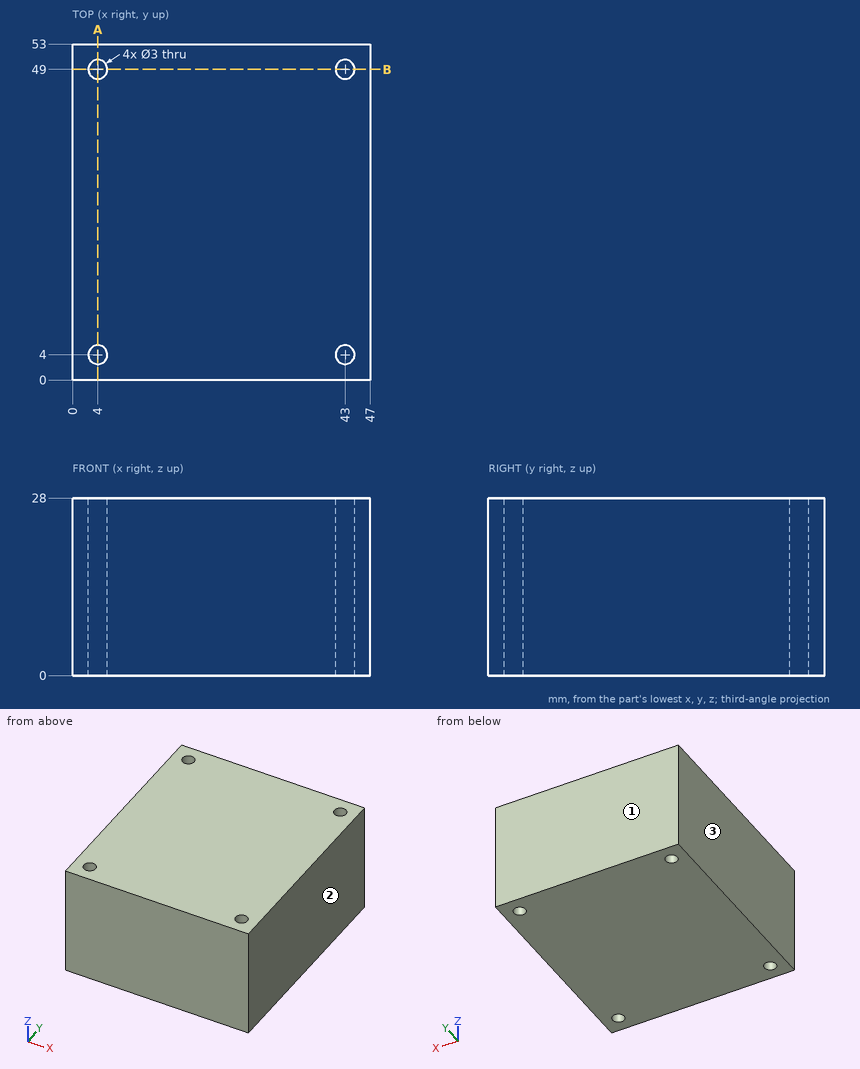
The figure shows three views and two pictorial views of one solid part (mm, origin at its lowest corner). Answer the questions. Give positions to 0.01 mm unless a question says otherwise; leave off trailing zeros. Write each loop counter-clockwise with the first axis right and the second up, starting at its lowest first coordinate (ties: lowest second). Pieces come first, ordered by that corner, then holes. Notation, with made-up numbers: (57, -5) - (85, -5) arc R21 cw to (85, 13) - close; hole circle Ø1 at (17.5, 18). An arc over 180 degrees is marked (long way). Use CSV: the item, a comma, the result in double quotes. Start each with the question number.
Item 1: The mould has two halves that part along X. Classify the marked faces 1, 2 and 3: pulls with the +X half, pulls with the -X half, needs draft (parallel to the pull), parting line crosses it, or undercut.
Item 2: The part is cut by section A-A, the plane x = 4. Give the vertices of the cut face in (y, z).
Item 3: The part is cut by section B-B, the plane y = 49. Give the vertices of the cut face in (x, z), and give its area (3 significant figures).
Item 4: Consider line 1 (Y direction, x = 4, z = 20.25); line 2 (X direction, y = 4, z = 6.5); line 3 (X direction, y = 5, z = 20.25). Determine where each line is inside the solid, lowest interval first.
Taken from the geometry:
1,face 1,"needs draft"
1,face 2,"pulls with the +X half"
1,face 3,"pulls with the -X half"
2,outline,"(0, 0) - (2.5, 0) - (2.5, 28) - (0, 28) - close; (5.5, 0) - (47.5, 0) - (47.5, 28) - (5.5, 28) - close; (50.5, 0) - (53, 0) - (53, 28) - (50.5, 28) - close"
3,outline,"(0, 0) - (2.5, 0) - (2.5, 28) - (0, 28) - close; (5.5, 0) - (41.5, 0) - (41.5, 28) - (5.5, 28) - close; (44.5, 0) - (47, 0) - (47, 28) - (44.5, 28) - close"
3,area,"1,150 mm2"
4,line 1,"0 to 2.5, 5.5 to 47.5, 50.5 to 53"
4,line 2,"0 to 2.5, 5.5 to 41.5, 44.5 to 47"
4,line 3,"0 to 2.88, 5.12 to 41.88, 44.12 to 47"
